```python
from build123d import *

# Parameters (mm, degrees)
BASE_SKETCH_R                                      = 62.5
BOSS_EXTRUDE1_DEPTH                                = 10
BOSS_EXTRUDE2_START                                = -10
BASE_SKETCH_3_R                                    = 10
BASE_SKETCH_3_R_2                                  = 5
BOSS_EXTRUDE2_DEPTH                                = 25
FILLET1_R                                          = 5
CHAMFER1_SIZE                                      = 2
CBORE_FOR_M2_5_HEX_HEAD_MACHINE_SCREW1_D           = 3.1
CBORE_FOR_M2_5_HEX_HEAD_MACHINE_SCREW1_CBORE_D     = 7.28
CBORE_FOR_M2_5_HEX_HEAD_MACHINE_SCREW1_CBORE_DEPTH = 2.1
CUT_EXTRUDE2_DEPTH                                 = 2.5


with BuildPart() as part:
    # Base_Sketch → Boss-Extrude1 (new body)
    with BuildSketch(Plane.XY):
        Circle(BASE_SKETCH_R)
    extrude(amount=-BOSS_EXTRUDE1_DEPTH)

    # Base_Sketch<3> → Boss-Extrude2 (add)
    with BuildSketch(Plane.XY.offset(BOSS_EXTRUDE2_START)):
        Circle(BASE_SKETCH_3_R)
        Circle(BASE_SKETCH_3_R_2, mode=Mode.SUBTRACT)
    extrude(amount=-BOSS_EXTRUDE2_DEPTH)

    # Fillet1
    fillet1_edges = [part.edges().sort_by_distance(p)[0] for p in [
        (-62.5, 0, -10),
        (-10, 0, -10),
    ]]
    fillet(fillet1_edges, radius=FILLET1_R)

    # Chamfer1
    chamfer1_edges = [part.edges().sort_by_distance(p)[0] for p in [
        (-10, 0, -35),
    ]]
    chamfer(chamfer1_edges, length=CHAMFER1_SIZE)

    # CBORE for M2.5 Hex Head Machine Screw1 (through all)
    with Locations(Plane(origin=(0, 10, -25), x_dir=(1, 0, 0), z_dir=(0, 1, 0))):
        with Locations((0, 0)):
            CounterBoreHole(CBORE_FOR_M2_5_HEX_HEAD_MACHINE_SCREW1_D / 2, CBORE_FOR_M2_5_HEX_HEAD_MACHINE_SCREW1_CBORE_D / 2, CBORE_FOR_M2_5_HEX_HEAD_MACHINE_SCREW1_CBORE_DEPTH)

    # Nut_Extrude → Cut-Extrude2 (cut)
    with BuildSketch(Plane(origin=(0, -10, -35), x_dir=(-1, 0, 0), z_dir=(0, -1, 0))):
        Polygon((2.875, -11.659882024), (2.875, -8.340117976), (0, -6.680235952), (-2.875, -8.340117976), (-2.875, -11.659882024), (0, -13.319764048), align=None)
    extrude(amount=-CUT_EXTRUDE2_DEPTH, mode=Mode.SUBTRACT)


solid = part.part
```
Can you work these out from the model? Positions are in its coordinate system, mm. A direction names the side the tool comes from. Round coordinates to 2 decimals unless told otherwise and drop trailing zeros. Loops run counter-clockwise (first coordinate to the right, second up) from the corner with the lowest first, then second, coordinate; pieces in that order, holes last. Notation, with made-up numbers: (18.5, 49) -> (61.5, 49) arc R31 cw to (61.5, 84) -> close; hole circle Ø9 at (47, 23.25). An arc over 180 degrees is marked (long way). Answer in a Markdown table with one row per item.
Item 1: We'd pull the mould along Z, two halves only. Please class faces 4 (the flat face through (1.3, -7.5, -23.6)), 5 (the flat face through (0, 0, -10)), 6 (the cylindrical face through (-62.44, 2.75, -2.46)), 7 (the cylindrical face through (1.55, 6.3, -25.07)): released by +Z, released by -Z, zero draft, split by the parting line, or undercut.
Answer block:
| item | result |
|---|---|
| face 4 | undercut |
| face 5 | released by -Z |
| face 6 | zero draft |
| face 7 | undercut |
Item 2: Suppose I cut it at A-A, the plane z = -25. List the corners of the cut face in (x, y) for me (3 decimals), plus the area to 3 significant figures.
Answer block:
| item | result |
|---|---|
| outline | (-3.64, 7.9) -> (-3.64, 9.314) arc R10 ccw to (-2.875, -9.578) -> (-2.875, -7.5) -> (-1.55, -7.5) -> (-1.55, -4.754) arc R5 cw to (-1.55, 4.754) -> (-1.55, 7.9) -> close; (1.55, -7.5) -> (2.875, -7.5) -> (2.875, -9.578) arc R10 ccw to (3.64, 9.314) -> (3.64, 7.9) -> (1.55, 7.9) -> (1.55, 4.754) arc R5 cw to (1.55, -4.754) -> close |
| area | 191 mm² |
Item 3: If I drill on probe 1 along Z at (x, y) = (0, -6.9); probe 2 along X at (y, z) = (-6, -25); probe 3 along Z at (x, y) = (54, 1), over which ranges is the centre line in solid material (lowest first)?
Answer block:
| item | result |
|---|---|
| probe 1 | -35 to -26.55, -23.45 to 0 |
| probe 2 | -8 to -1.55, 1.55 to 8 |
| probe 3 | -10 to 0 |
Item 4: Will these pins go through, and if not, where does the flat tip stop? P1, Ø3.5, axis at x = -1.5, z = -25, coming from the +Y side; P2, Ø6, axis at x = 0, y = 0, coming from the -Z side; P3, Ø0.6, axis at y = -9, z = -25.5, coming from the -X side; P4, Ø2.5, axis at x = 0, z = -25, coming from the -Y side.
Answer block:
| item | result |
|---|---|
| P1 | y = 7.9 |
| P2 | z = -10 |
| P3 | x = -4.93 |
| P4 | through |
Item 5: On a 3-axis mill with a long thin cutter (end or side, diameter ignored), from which of +Z, -Z, +X, -X, +Y, -Y can I reach the whole of each face in a straight line? I mean faces 1 (the cylindrical face through (-3.636, 8.733, -25.16)), 2 (the cylindrical face through (4.77, 1.5, -22.32)), 3 (the cylindrical face through (1.55, -6.14, -25.07)). Say none if no direction works.
Answer block:
| item | result |
|---|---|
| face 1 | +Y |
| face 2 | -Z |
| face 3 | +Y, -Y |
Item 6: Suppose I cut it at D-D, the plane z = -2. List the corners of the cut face in (x, y) for me.
Answer block:
| item | result |
|---|---|
| outline | circle Ø125 at (0, 0) |
Item 7: Suppose I cut it at C-C, the plane z = -12. List the corners of the cut face in (x, y) for me.
Answer block:
| item | result |
|---|---|
| outline | circle Ø22 at (0, 0); hole circle Ø10 at (0, 0) |
Item 8: Suppose I cut it at B-B, the plane y = 0. List the corners of the cut face in (x, z) for me.
Answer block:
| item | result |
|---|---|
| outline | (-62.5, -5) arc R5 ccw to (-57.5, -10) -> (-15, -10) arc R5 cw to (-10, -15) -> (-10, -33) -> (-8, -35) -> (-5, -35) -> (-5, -10) -> (5, -10) -> (5, -35) -> (8, -35) -> (10, -33) -> (10, -15) arc R5 cw to (15, -10) -> (57.5, -10) arc R5 ccw to (62.5, -5) -> (62.5, 0) -> (-62.5, 0) -> close |
